The model under review builds one solid part; all positions refer to its coordinate system, in mm. Give positions to 0.01 mm unless a question says otherwise; leave off trailing zeros. Write each loop counter-clockwise with the first axis right and the second up, starting at its lowest first coordinate (ties: lowest second). Pieces come first, ordered by that corner, then holes. Notation, with made-up numbers: (86.5, -8) - (109.5, -8) arc R21 cw to (109.5, 17) - close; hole circle Ø11 at (66.25, 19.5). An arc over 180 degrees is marked (long way). Write item = value, one per line.
```python
from build123d import *

# Parameters (mm, degrees)
F0_R     = 10.6
F1_DEPTH = 5
F0_R_2   = 8.1
F2_DEPTH = 5


# Not quite as in the source:
# - ends of sketch curves that miss each other by under 0.0002 mm in the source are joined


with BuildPart() as f1:
    # F0 (on Top) → F1 (new body)
    with BuildSketch(Plane.XY):
        with BuildLine():
            ThreePointArc((27.8263414504, 16.9481692723), (16.199467196, 28.0319950031), (0.7904601582, 32.5704859273))
            ThreePointArc((0.7904601582, 32.5704859273), (7.7697772708, 29.2104480555), (10.6, 22))
            ThreePointArc((10.6, 22), (-7.2200130901, 14.2391101684), (-0.7644171658, 32.5724011651))
            ThreePointArc((-0.7644171658, 32.5724011651), (-16.1766867062, 28.0451473253), (-27.8116156006, 16.9698365243))
            ThreePointArc((-27.8116156006, 16.9698365243), (-15.9289393792, 21.1293147465), (-8.4525595083, 11.0000009845))
            ThreePointArc((-8.4525595083, 11.0000009845), (-21.4248089079, 0.6688619967), (-28.5907543736, 15.6241591469))
            ThreePointArc((-28.5907543736, 15.6241591469), (-32.3761533963, 0.0131339969), (-28.6021197402, -15.6006426749))
            ThreePointArc((-28.6021197402, -15.6006426749), (-21.4120811641, -0.665945501), (-8.4525606734, -10.9999990645))
            ThreePointArc((-8.4525606734, -10.9999990645), (-15.9414195658, -21.1331526215), (-27.8262967127, -16.9482387968))
            ThreePointArc((-27.8262967127, -16.9482387968), (-16.1994359735, -28.0320130446), (-0.7904706999, -32.5704854113))
            ThreePointArc((-0.7904706999, -32.5704854113), (-7.2104473679, -14.2302200266), (10.5999976698, -22.0000000981))
            ThreePointArc((10.5999976698, -22.0000000981), (7.7608872989, -29.2200134059), (0.7644142424, -32.5724013061))
            ThreePointArc((0.7644142424, -32.5724013061), (16.17671692, -28.045129896), (27.8116549786, -16.9697754267))
            ThreePointArc((27.8116549786, -16.9697754267), (8.9232325044, -7.8764163379), (29.652557178, -11.0000010826))
            ThreePointArc((29.652557178, -11.0000010826), (29.3836867135, -13.3722916469), (28.5907151929, -15.6242352553))
            ThreePointArc((28.5907151929, -15.6242352553), (32.3761533958, -0.0131351765), (28.6020816932, 15.6007167134))
            ThreePointArc((28.6020816932, 15.6007167134), (29.3866027477, 13.3595595706), (29.6525583432, 10.9999989665))
            ThreePointArc((29.6525583432, 10.9999989665), (8.9193924771, 7.8888979505), (27.8263414504, 16.9481692723))
        make_face()
        Circle(F0_R, mode=Mode.SUBTRACT)
    extrude(amount=F1_DEPTH)

    # F0 (on Top) → F2 (join)
    with BuildSketch(Plane.XY):
        with BuildLine():
            ThreePointArc((28.2460392226, -16.2763527502), (28.4201387166, -15.9512250463), (28.5907151929, -15.6242352553))
            ThreePointArc((28.5907151929, -15.6242352553), (29.3836867135, -13.3722916469), (29.652557178, -11.0000010826))
            ThreePointArc((29.652557178, -11.0000010826), (8.9232325044, -7.8764163379), (27.8116549786, -16.9697754267))
            ThreePointArc((27.8116549786, -16.9697754267), (28.023981709, -16.6361065668), (28.2324281634, -16.3))
            ThreePointArc((28.2324281634, -16.3), (28.2392409163, -16.2881805324), (28.2460392226, -16.2763527502))
        make_face()
        with Locations((19.052557178, -11.0000010826)):
            Circle(F0_R_2, mode=Mode.SUBTRACT)
        with BuildLine():
            ThreePointArc((28.2187545739, 16.3236111479), (28.0242350806, 16.636950204), (27.8263414504, 16.9481692723))
            ThreePointArc((27.8263414504, 16.9481692723), (8.9193924771, 7.8888979505), (29.6525583432, 10.9999989665))
            ThreePointArc((29.6525583432, 10.9999989665), (29.3866027477, 13.3595595706), (28.6020816932, 15.6007167134))
            ThreePointArc((28.6020816932, 15.6007167134), (28.4192805282, 15.9514291247), (28.2324281634, 16.3))
            ThreePointArc((28.2324281634, 16.3), (28.2255985395, 16.3118097271), (28.2187545739, 16.3236111479))
        make_face()
        with Locations((19.0525583432, 10.9999989665)):
            Circle(F0_R_2, mode=Mode.SUBTRACT)
        with BuildLine():
            ThreePointArc((0.0272846487, -32.5999638982), (0.3959239022, -32.5881738584), (0.7644142424, -32.5724013061))
            ThreePointArc((0.7644142424, -32.5724013061), (7.7608872989, -29.2200134059), (10.5999976698, -22.0000000981))
            ThreePointArc((10.5999976698, -22.0000000981), (-7.2104473679, -14.2302200266), (-0.7904706999, -32.5704854113))
            ThreePointArc((-0.7904706999, -32.5704854113), (-0.3953208493, -32.5875325821), (0, -32.6))
            ThreePointArc((0, -32.6), (0.013642337, -32.5999913161), (0.0272846487, -32.5999638982))
        make_face()
        with Locations((-2.3302e-06, -22.0000000981)):
            Circle(F0_R_2, mode=Mode.SUBTRACT)
        Circle(F0_R)
        Circle(F0_R_2, mode=Mode.SUBTRACT)
        with BuildLine():
            ThreePointArc((-8.4525606734, -10.9999990645), (-21.4120811641, -0.665945501), (-28.6021197402, -15.6006426749))
            ThreePointArc((-28.6021197402, -15.6006426749), (-28.4192999794, -15.9513923284), (-28.2324281634, -16.3))
            ThreePointArc((-28.2324281634, -16.3), (-28.2256003271, -16.3118107622), (-28.218756359, -16.3236121847))
            ThreePointArc((-28.218756359, -16.3236121847), (-28.0242130887, -16.6369852059), (-27.8262967127, -16.9482387968))
            ThreePointArc((-27.8262967127, -16.9482387968), (-15.9414195658, -21.1331526215), (-8.4525606734, -10.9999990645))
        make_face()
        with Locations((-19.0525606734, -10.9999990645)):
            Circle(F0_R_2, mode=Mode.SUBTRACT)
        with BuildLine():
            ThreePointArc((-8.4525595083, 11.0000009845), (-15.9289393792, 21.1293147465), (-27.8116156006, 16.9698365243))
            ThreePointArc((-27.8116156006, 16.9698365243), (-28.0239623753, 16.6361373416), (-28.2324281634, 16.3))
            ThreePointArc((-28.2324281634, 16.3), (-28.2392426242, 16.2881815155), (-28.2460409731, 16.2763537548))
            ThreePointArc((-28.2460409731, 16.2763537548), (-28.420158717, 15.951187206), (-28.5907543736, 15.6241591469))
            ThreePointArc((-28.5907543736, 15.6241591469), (-21.4248089079, 0.6688619967), (-8.4525595083, 11.0000009845))
        make_face()
        with Locations((-19.0525595083, 11.0000009845)):
            Circle(F0_R_2, mode=Mode.SUBTRACT)
        with BuildLine():
            ThreePointArc((0.7904601582, 32.5704859273), (0.3953155758, 32.587532779), (0, 32.6))
            ThreePointArc((0, 32.6), (-0.0136423369, 32.5999912211), (-0.0272846512, 32.5999648843))
            ThreePointArc((-0.0272846512, 32.5999648843), (-0.3959253645, 32.5881738038), (-0.7644171658, 32.5724011651))
            ThreePointArc((-0.7644171658, 32.5724011651), (-7.2200130901, 14.2391101684), (10.6, 22))
            ThreePointArc((10.6, 22), (7.7697772708, 29.2104480555), (0.7904601582, 32.5704859273))
        make_face()
        with Locations((0, 22)):
            Circle(F0_R_2, mode=Mode.SUBTRACT)
    extrude(amount=F2_DEPTH)


solid = f1.part
```
1. Take a section at B-B on x = 22.5. Give the boundary of the cut face in (y, z), and give its area (3 significant figures).
Findings below:
outline = (-23.35, 0) - (-18.33, 0) - (-18.33, 5) - (-23.35, 5) - close; (-3.67, 0) - (3.67, 0) - (3.67, 5) - (-3.67, 5) - close; (18.33, 0) - (23.35, 0) - (23.35, 5) - (18.33, 5) - close
area = 86.9 mm²
2. Insertion check: P1, Ø13, axis at x = 19.05, y = -11, coming from the +Z side; P2, Ø3, axis at x = 8.5, z = 3, coming from the -Y side; P3, Ø2, axis at x = 8.5, z = 1.5, coming from the -Y side; P4, Ø2, axis at x = 23.5, z = 3, coming from the +Y side. Each pin has a flat end and moves straight along its axis. Give the tip position at first contact, or say it passes through.
Findings below:
P1 = through
P2 = -31.69
P3 = -31.57
P4 = 23.35
3. Take a section at C-C on z = 1.6. Count the separate pieces of the cut face and the enclosed holes in it, and give its area (3 significant figures).
Findings below:
separate_pieces = 1
enclosed_holes = 7
area = 1,870 mm²
4. Take a section at D-D on y = 20. Give the boundary of the cut face in (x, z).
Findings below:
outline = (-25.61, 0) - (-7.85, 0) - (-7.85, 5) - (-25.61, 5) - close; (7.85, 0) - (25.62, 0) - (25.62, 5) - (7.85, 5) - close
5. For line 1 (X direction, y = -17.5, z = 4.65); line 2 (Y direction, x = 17.5, z = 3.8); line 3 (Y direction, x = 7, z = 4.8), list the stretches that pass through material, from the lowest coordinate up. Write a range as from..to.
Findings below:
line_1 = -27.46..-23.89, -14.22..-6.73, 6.73..14.22, 23.89..27.46
line_2 = -27.24..-18.95, -3.05..3.05, 18.95..27.24
line_3 = -31.69..-26.08, -17.92..-4.08, 4.08..17.92, 26.08..31.69
6. Take a section at A-A on y = 0. Give the boundary of the cut face in (x, z), and give its area (3 significant figures).
Findings below:
outline = (-32.38, 0) - (-8.1, 0) - (-8.1, 5) - (-32.38, 5) - close; (8.1, 0) - (32.38, 0) - (32.38, 5) - (8.1, 5) - close
area = 243 mm²
